```python
from build123d import *

# Parameters (mm, degrees)
BOSS_EXTRUDE1_DEPTH     = 5
CUT_EXTRUDE1_DEPTH      = 26.951878545
CUT_EXTRUDE1_DEPTH_BACK = 26.951878545
SKETCH4_W               = 1.55
SKETCH4_H               = 10


with BuildPart() as part:
    # Sketch2 → Revolve1 (revolve)
    with BuildSketch(Plane.XY):
        Polygon((0, 0), (8.5, 0), (8.5, 7), (3.5, 7), (3.5, 13), (3, 13), (3, 23), (0, 23), align=None)
    revolve(axis=Axis((0, -1000, 0), (0, 1, 0)))

    # Sketch3 → Boss-Extrude1 (add)
    with BuildSketch(Plane.XZ):
        with BuildLine():
            Line((6.544190201, 4.773214286), (6.786567616, 4.95))
            ThreePointArc((6.786567616, 4.95), (7.327590965, 4.106873586), (7.76439466, 3.205335485))
            Line((7.76439466, 3.205335485), (7.48709485, 3.090859217))
            ThreePointArc((7.48709485, 3.090859217), (7.065891288, 3.960199529), (6.544190201, 4.773214286))
        make_face()
        with BuildLine():
            Line((8.042397221, 0.964285714), (8.340263785, 1))
            ThreePointArc((8.340263785, 1), (8.4, 0), (8.340263785, -1))
            Line((8.340263785, -1), (8.042397221, -0.964285714))
            ThreePointArc((8.042397221, -0.964285714), (8.1, 0), (8.042397221, 0.964285714))
        make_face()
        with BuildLine():
            Line((7.48709485, -3.090859217), (7.76439466, -3.205335485))
            ThreePointArc((7.76439466, -3.205335485), (7.327590965, -4.106873586), (6.786567616, -4.95))
            Line((6.786567616, -4.95), (6.544190201, -4.773214286))
            ThreePointArc((6.544190201, -4.773214286), (7.065891288, -3.960199529), (7.48709485, -3.090859217))
        make_face()
        with BuildLine():
            Line((-1.928571429, -7.867058678), (-2, -8.158431222))
            ThreePointArc((-2, -8.158431222), (0, -8.4), (2, -8.158431222))
            Line((2, -8.158431222), (1.928571429, -7.867058678))
            ThreePointArc((1.928571429, -7.867058678), (0, -8.1), (-1.928571429, -7.867058678))
        make_face()
        with BuildLine():
            Line((-1.928571429, 7.867058678), (-2, 8.158431222))
            ThreePointArc((-2, 8.158431222), (0, 8.4), (2, 8.158431222))
            Line((2, 8.158431222), (1.928571429, 7.867058678))
            ThreePointArc((1.928571429, 7.867058678), (0, 8.1), (-1.928571429, 7.867058678))
        make_face()
    extrude(amount=BOSS_EXTRUDE1_DEPTH)

    # Sketch4 → Cut-Extrude1 (cut, two sides: drawn at the far end of the back side and taken through both)
    with BuildSketch(Plane(origin=(0, 0, 0), x_dir=(0, 0, -1), z_dir=(1, 0, 0)).offset(-CUT_EXTRUDE1_DEPTH_BACK)):
        with Locations((2.225, 18)):
            Rectangle(SKETCH4_W, SKETCH4_H)
    extrude(amount=CUT_EXTRUDE1_DEPTH + CUT_EXTRUDE1_DEPTH_BACK, mode=Mode.SUBTRACT)


solid = part.part
```
Read the model definition and answer for the solid it produces. Units are mm, in the model's axes. A direction names the side the tool comes from. Round coordinates to 2 decimals unless told otherwise and drop trailing zeros. Write each loop counter-clockwise with the first axis right and the second up, starting at its lowest first coordinate (ties: lowest second). Pieces come first, ordered by that corner, then holes. Notation, with made-up numbers: (12.5, 81.5) -> (40.5, 81.5) arc R20 ccw to (40.5, 108.5) -> close; hole circle Ø6 at (5.5, -38). An arc over 180 degrees is marked (long way). Answer in a Markdown table with one row per item. Add a question column.
1) Find section A-A, the plane z = 0. Determine the outline of the cut face in (x, y).
2) Given P1, Ø5, axis at x = 4, y = 10.5, coming from the -Z side; P2, Ø6, axis at x = -2, z = 2, coming from the -Y side; P3, Ø2.5, axis at x = 1, y = 16, coming from the -Z side, each flat-ended and moving along its own axis, determine where each tip first touches the part or whether it passes through.
3) Which of the six approach directions +Z, -Z, +X, -X, +Y, -Y give full straight-line access (tool end or side, diameter ignored) to faces 4 (the face through (7.334, -2.465, -4.095)), 5 (the face through (0, -2.5, 8.1)), 6 (the face through (8.1, -2.5, 0)), 7 (the face through (0, 13, -2)), 8 (the face through (0, 18, -1.45))?
4) Find section C-C, the plane y = 0.75. Determine the outline of the cut face in (x, z).
5) Find section D-D, the plane x = 5. Determine the outline of the cut face in (y, z).
6) Determine the mould class of faces 1 (the face through (0, 23, 0)), 2 (the face through (0, -2.5, -8.1)), 3 (the face through (3.233, 10.042, 1.341)) for opening direction X: pulls with the +X half, pulls with the -X half, needs draft (parallel to the pull), parting line crosses it, or undercut.
7) Find section B-B, the plane x = 0. Determine the outline of the cut face in (y, z), and give its area (4 significant figures).
8) Consider line 1 (Y direction, x = -7, z = -3.75); line 2 (Z direction, x = -6.75, y = 6.5); line 3 (Z direction, x = -1.5, y = 8.5). Determine where each line is inside the solid, lowest interval first.
Findings below:
| question | item | result |
|---|---|---|
| 1 | outline | (-8.5, 0) -> (8.1, 0) -> (8.1, -5) -> (8.4, -5) -> (8.4, 0) -> (8.5, 0) -> (8.5, 7) -> (3.5, 7) -> (3.5, 13) -> (3, 13) -> (3, 23) -> (-3, 23) -> (-3, 13) -> (-3.5, 13) -> (-3.5, 7) -> (-8.5, 7) -> close |
| 2 | P1 | z = -3.16 |
| 2 | P2 | y = 0 |
| 2 | P3 | z = -1.45 |
| 3 | face 4 | -Z, +X, -Y |
| 3 | face 5 | -Y |
| 3 | face 6 | -X, -Y |
| 3 | face 7 | +Y |
| 3 | face 8 | -Z, +X, -X, +Y |
| 4 | outline | circle Ø17 at (0, 0) |
| 5 | outline | (0, -6.87) -> (7, -6.87) -> (7, 6.87) -> (0, 6.87) -> close |
| 6 | face 1 | needs draft |
| 6 | face 2 | undercut |
| 6 | face 3 | parting line crosses it |
| 7 | outline | (-5, -8.4) -> (0, -8.4) -> (0, -8.5) -> (7, -8.5) -> (7, -3.5) -> (13, -3.5) -> (13, -1.45) -> (23, -1.45) -> (23, 3) -> (13, 3) -> (13, 3.5) -> (7, 3.5) -> (7, 8.5) -> (0, 8.5) -> (0, 8.4) -> (-5, 8.4) -> (-5, 8.1) -> (0, 8.1) -> (0, -8.1) -> (-5, -8.1) -> close |
| 7 | area | 208.5 mm² |
| 8 | line 1 | 0 to 7 |
| 8 | line 2 | -5.17 to 5.17 |
| 8 | line 3 | -3.16 to 3.16 |
